from build123d import *

# Parameters (mm, degrees)
CROQUIS1_W              = 220
CROQUIS1_H              = 480
SALIENTE_EXTRUIR1_DEPTH = 3
CROQUIS2_R              = 5
CORTAR_EXTRUIR1_DEPTH   = 3


with BuildPart() as part:
    # Croquis1 → Saliente-Extruir1 (new body)
    with BuildSketch(Plane.XY):
        Rectangle(CROQUIS1_W, CROQUIS1_H)
    extrude(amount=SALIENTE_EXTRUIR1_DEPTH)

    # Croquis2 → Cortar-Extruir1 (cut)
    with BuildSketch(Plane(origin=(0, 0, 0), x_dir=(-1, 0, 0), z_dir=(0, 0, -1))):
        with Locations((-80, 215)):
            Circle(CROQUIS2_R)
        with Locations((80, 215)):
            Circle(CROQUIS2_R)
        with Locations((80, -215)):
            Circle(CROQUIS2_R)
        with Locations((-80, -215)):
            Circle(CROQUIS2_R)
        with BuildLine():
            Line((-100, 3.25), (-50, 3.25))
            ThreePointArc((-50, 3.25), (-46.75, 0), (-50, -3.25))
            Line((-50, -3.25), (-100, -3.25))
            ThreePointArc((-100, -3.25), (-103.25, 0), (-100, 3.25))
        make_face()
        with BuildLine():
            Line((-100, 93.25), (-50, 93.25))
            ThreePointArc((-50, 93.25), (-46.75, 90), (-50, 86.75))
            Line((-50, 86.75), (-100, 86.75))
            ThreePointArc((-100, 86.75), (-103.25, 90), (-100, 93.25))
        make_face()
        with BuildLine():
            Line((-100, -93.25), (-50, -93.25))
            ThreePointArc((-50, -93.25), (-46.75, -90), (-50, -86.75))
            Line((-50, -86.75), (-100, -86.75))
            ThreePointArc((-100, -86.75), (-103.25, -90), (-100, -93.25))
        make_face()
        with BuildLine():
            Line((-25, 3.25), (25, 3.25))
            ThreePointArc((25, 3.25), (28.25, 0), (25, -3.25))
            Line((25, -3.25), (-25, -3.25))
            ThreePointArc((-25, -3.25), (-28.25, 0), (-25, 3.25))
        make_face()
        with BuildLine():
            Line((-25, 93.25), (25, 93.25))
            ThreePointArc((25, 93.25), (28.25, 90), (25, 86.75))
            Line((25, 86.75), (-25, 86.75))
            ThreePointArc((-25, 86.75), (-28.25, 90), (-25, 93.25))
        make_face()
        with BuildLine():
            Line((-25, -93.25), (25, -93.25))
            ThreePointArc((25, -93.25), (28.25, -90), (25, -86.75))
            Line((25, -86.75), (-25, -86.75))
            ThreePointArc((-25, -86.75), (-28.25, -90), (-25, -93.25))
        make_face()
        with BuildLine():
            Line((50, 3.25), (100, 3.25))
            ThreePointArc((100, 3.25), (103.25, 0), (100, -3.25))
            Line((100, -3.25), (50, -3.25))
            ThreePointArc((50, -3.25), (46.75, 0), (50, 3.25))
        make_face()
        with BuildLine():
            Line((50, 93.25), (100, 93.25))
            ThreePointArc((100, 93.25), (103.25, 90), (100, 86.75))
            Line((100, 86.75), (50, 86.75))
            ThreePointArc((50, 86.75), (46.75, 90), (50, 93.25))
        make_face()
        with BuildLine():
            Line((50, -93.25), (100, -93.25))
            ThreePointArc((100, -93.25), (103.25, -90), (100, -86.75))
            Line((100, -86.75), (50, -86.75))
            ThreePointArc((50, -86.75), (46.75, -90), (50, -93.25))
        make_face()
        with BuildLine():
            Line((-100, 183.25), (-50, 183.25))
            ThreePointArc((-50, 183.25), (-46.75, 180), (-50, 176.75))
            Line((-50, 176.75), (-100, 176.75))
            ThreePointArc((-100, 176.75), (-103.25, 180), (-100, 183.25))
        make_face()
        with BuildLine():
            Line((-25, 183.25), (25, 183.25))
            ThreePointArc((25, 183.25), (28.25, 180), (25, 176.75))
            Line((25, 176.75), (-25, 176.75))
            ThreePointArc((-25, 176.75), (-28.25, 180), (-25, 183.25))
        make_face()
        with BuildLine():
            Line((50, 183.25), (100, 183.25))
            ThreePointArc((100, 183.25), (103.25, 180), (100, 176.75))
            Line((100, 176.75), (50, 176.75))
            ThreePointArc((50, 176.75), (46.75, 180), (50, 183.25))
        make_face()
        with BuildLine():
            Line((-100, -183.25), (-50, -183.25))
            ThreePointArc((-50, -183.25), (-46.75, -180), (-50, -176.75))
            Line((-50, -176.75), (-100, -176.75))
            ThreePointArc((-100, -176.75), (-103.25, -180), (-100, -183.25))
        make_face()
        with BuildLine():
            Line((-25, -183.25), (25, -183.25))
            ThreePointArc((25, -183.25), (28.25, -180), (25, -176.75))
            Line((25, -176.75), (-25, -176.75))
            ThreePointArc((-25, -176.75), (-28.25, -180), (-25, -183.25))
        make_face()
        with BuildLine():
            Line((50, -183.25), (100, -183.25))
            ThreePointArc((100, -183.25), (103.25, -180), (100, -176.75))
            Line((100, -176.75), (50, -176.75))
            ThreePointArc((50, -176.75), (46.75, -180), (50, -183.25))
        make_face()
    extrude(amount=-CORTAR_EXTRUIR1_DEPTH, mode=Mode.SUBTRACT)


solid = part.part
The model under review builds one solid part; all positions refer to its coordinate system, in mm. Coordinates: 2 decimals unless noted, no trailing zeros. Loops run counter-clockwise (first coordinate to the right, second up) from the corner with the lowest first, then second, coordinate; pieces in that order, holes last. Notation, with made-up numbers: (3.5, -16.5) -> (52.5, -16.5) arc R19 ccw to (52.5, 15.5) -> close; hole circle Ø10 at (40, -3.5). An arc over 180 degrees is marked (long way). Use a Markdown table: item, result. Add a question column.
1. Add section A-A on x = -80. Give the number of separate pieces and of enclosed holes in the cut face, plus the area to 3 significant figures.
2. To check wall thickness, follow line 1 (Y direction, x = -91, z = 2.85). State the ranges of the line that lie inside material, in increasing order.
3. Draft analysis for pull direction Y (two halves, no side actions). For faces 1 (the face through (-26, 3.4, 0)), 2 (the face through (77, -211, 1)), state which applies: pulls with the +Y half, pulls with the -Y half, needs draft (parallel to the pull), parting line crosses it, or undercut.
4. Add section B-B on x = 6. Write out the cut boundary in (y, z), plus the area to 3 significant figures.
Returned:
| question | item | result |
|---|---|---|
| 1 | separate pieces | 8 |
| 1 | enclosed holes | 0 |
| 1 | area | 1,280 mm² |
| 2 | line 1 | y = -240 to -183.25, -176.75 to -93.25, -86.75 to -3.25, 3.25 to 86.75, 93.25 to 176.75, 183.25 to 240 |
| 3 | face 1 | needs draft |
| 3 | face 2 | undercut |
| 4 | outline | (-240, 0) -> (-183.25, 0) -> (-183.25, 3) -> (-240, 3) -> close; (-176.75, 0) -> (-93.25, 0) -> (-93.25, 3) -> (-176.75, 3) -> close; (-86.75, 0) -> (-3.25, 0) -> (-3.25, 3) -> (-86.75, 3) -> close; (3.25, 0) -> (86.75, 0) -> (86.75, 3) -> (3.25, 3) -> close; (93.25, 0) -> (176.75, 0) -> (176.75, 3) -> (93.25, 3) -> close; (183.25, 0) -> (240, 0) -> (240, 3) -> (183.25, 3) -> close |
| 4 | area | 1,340 mm² |
